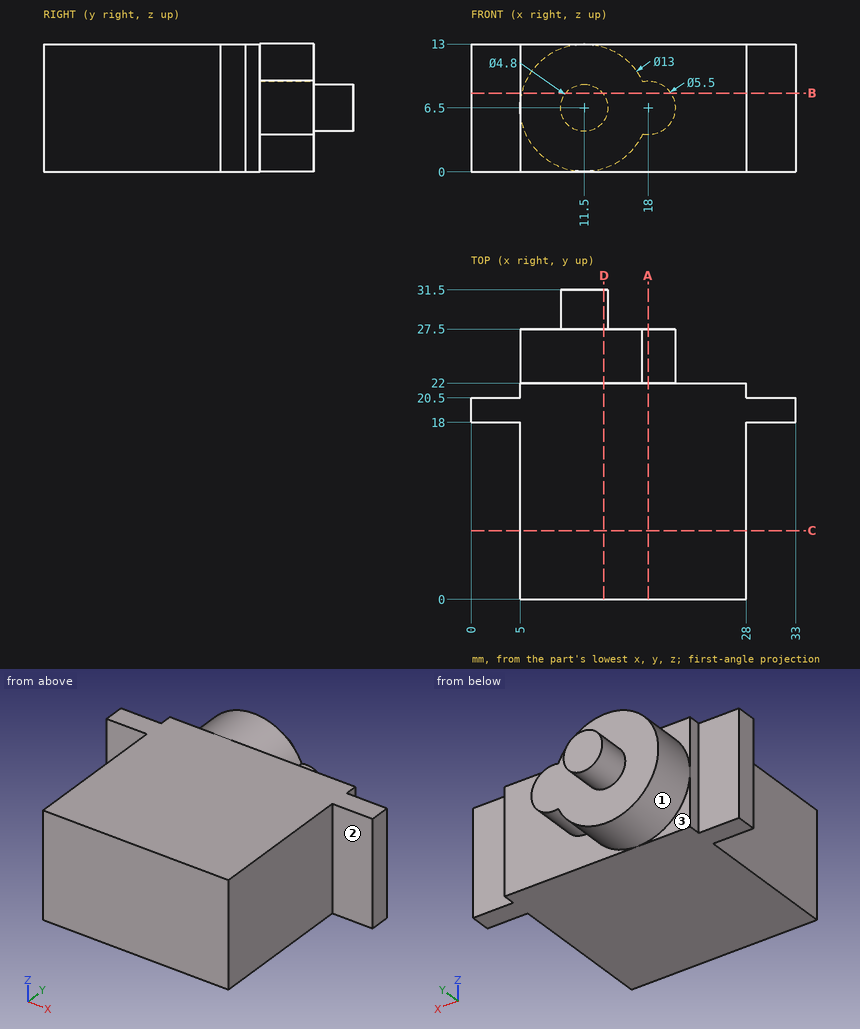
Could you check a few things on this drawing? It's one solid part, dimensions in mm from its lowest x, y, z. A direction names the side the tool comes from. Give positions to 0.01 mm unless a question says otherwise; leave off trailing zeros. Order: outer loops, then holes, each group sorted by start corner. A loop starts at its lowest first (then second) coordinate and runs counter-clockwise, first axis right, second up. Notation, with made-up numbers: (42.25, 89.5) - (100.25, 89.5) arc R15 cw to (100.25, 95.5) - close; hole circle Ø8 at (-20.75, -39.75). An arc over 180 degrees is marked (long way). One line per item, written item: value. Start each with the question number.
1. If I drill on probe 1 along Y at (x, z) = (8, 11); probe 2 along Y at (x, z) = (20, 11.5); probe 3 along X at (y, z) = (4.5, 2.5), over which ranges is the centre line in solid material (lowest first)?
2. Imagine slicing it at C-C on y = 7. List the corners of the cut face in (x, z) for me, plus the area to 3 significant figures.
3. For P1, Ø0.8, axis at y = 21.5, z = 7, coming from the +X side; P2, Ø2.5, axis at x = 31, z = 7.5, coming from the -Y side; P3, Ø6.5, axis at y = 13.5, z = 7.5, coming from the -X side, each with a flat end and sliding along its axis, tell me the tip position at first contact or that it passes through.
4. Imagine slicing it at B-B on z = 8. List the corners of the cut face in (x, y) for me.
5. For the marked faces 1, 2 and 3, which set-ups out of +Z, -Z, +X, -X, +Y, -Y let a thin tool reach every point of the face, with its end or its side?
6. Imagine slicing it at A-A on x = 18. List the corners of the cut face in (y, z) for me, plus the area to 3 significant figures.
7. Imagine slicing it at D-D on x = 13.5. List the corners of the cut face in (y, z) for me.
Values:
1. probe 1: 0 to 27.5
1. probe 2: 0 to 22
1. probe 3: 5 to 28
2. outline: (5, 0) - (28, 0) - (28, 13) - (5, 13) - close
2. area: 299 mm²
3. P1: x = 28
3. P2: y = 18
3. P3: x = 5
4. outline: (0, 18) - (5, 18) - (5, 0) - (28, 0) - (28, 18) - (33, 18) - (33, 20.5) - (28, 20.5) - (28, 22) - (20.3, 22) - (20.3, 27.5) - (13.37, 27.5) - (13.37, 31.5) - (9.63, 31.5) - (9.63, 27.5) - (5.18, 27.5) - (5.18, 22) - (5, 22) - (5, 20.5) - (0, 20.5) - close
5. face 1: +Y
5. face 2: +Z, -Z, +X, -Y
5. face 3: -Z, -X, +Y
6. outline: (0, 0) - (22, 0) - (22, 3.75) - (27.5, 3.75) - (27.5, 9.25) - (22, 9.25) - (22, 13) - (0, 13) - close
6. area: 316 mm²
7. outline: (0, 0) - (22, 0) - (22, 0.32) - (27.5, 0.32) - (27.5, 5.17) - (31.5, 5.17) - (31.5, 7.83) - (27.5, 7.83) - (27.5, 12.68) - (22, 12.68) - (22, 13) - (0, 13) - close
